from build123d import *

# Parameters (mm, degrees)
SKETCH2_R           = 1.725
SKETCH2_W           = 10
SKETCH2_H           = 20
BOSS_EXTRUDE1_DEPTH = 1.55
FILLET1_R           = 1


with BuildPart() as part:
    # Sketch2 → Boss-Extrude1 (new body)
    # profile 1 of 4: a face of its own
    with BuildSketch(Plane(origin=(0, 0, 0), x_dir=(1, 0, 0), z_dir=(0, 1, 0))):
        Polygon((17.906706977, 15.176380902), (-1.411809549, 10), (-4, 19.659258263), (15.318516526, 24.835639165), align=None)
        with Locations(Location((11.78298262, 18.711914808, 0), (0, 0, 90))):
            Circle(SKETCH2_R, mode=Mode.SUBTRACT)
        with Locations(Location((2.123724357, 16.123724357, 0), (0, 0, 90))):
            Circle(SKETCH2_R, mode=Mode.SUBTRACT)
    # profile 2 of 4: a face of its own
    with BuildSketch(Plane(origin=(0, 0, 0), x_dir=(1, 0, 0), z_dir=(0, 1, 0))):
        Polygon((-1.411809549, 10), (-4, 19.659258263), (-5, 19.39130907), (-5, 10), align=None)
    # profile 3 of 4: a face of its own
    with BuildSketch(Plane(origin=(0, 0, 0), x_dir=(1, 0, 0), z_dir=(0, 1, 0))):
        Rectangle(SKETCH2_W, SKETCH2_H)
        with Locations(Location((0, 5, 0), (0, 0, 90))):
            Circle(SKETCH2_R, mode=Mode.SUBTRACT)
        with Locations(Location((0, -5, 0), (0, 0, 90))):
            Circle(SKETCH2_R, mode=Mode.SUBTRACT)
    # profile 4 of 4: a face of its own
    with BuildSketch(Plane(origin=(0, 0, 0), x_dir=(1, 0, 0), z_dir=(0, 1, 0))):
        Polygon((5, 11.718039191), (-1.411809549, 10), (5, 10), align=None)
    extrude(amount=BOSS_EXTRUDE1_DEPTH)

    # Fillet1
    fillet1_edges = [part.edges().sort_by_distance(p)[0] for p in [
        (-5, 0.775, 10),
        (-5, 0.775, -19.39130907),
        (15.318516526, 0.775, -24.835639165),
        (17.906706977, 0.775, -15.176380902),
        (5, 0.775, -11.718039191),
        (5, 0.775, 10),
    ]]
    fillet(fillet1_edges, radius=FILLET1_R)


solid = part.part
The listing builds one solid part. Answer for the finished solid, in the listing's coordinates (mm). A direction names the side the tool comes from. Give positions to 0.01 mm unless a question says otherwise; leave off trailing zeros. Loops run counter-clockwise (first coordinate to the right, second up) from the corner with the lowest first, then second, coordinate; pieces in that order, holes last. Notation, with made-up numbers: (51.25, 67.5) - (89.25, 67.5) arc R18 ccw to (89.25, 94.5) - close; hole circle Ø9 at (16, 73). An arc over 180 degrees is marked (long way). Use one line per item in the form item = value.
1. Section C-C on x = 2.5 is taken. Give the vertices of the cut face in (y, z).
Calculated:
outline = (0, -21.4) - (1.55, -21.4) - (1.55, -17.81) - (0, -17.81) - close; (0, -14.44) - (1.55, -14.44) - (1.55, 10) - (0, 10) - close
2. Section B-B on x = 0 is taken. Give the vertices of the cut face in (y, z) (3 decimals).
Calculated:
outline = (0, -20.731) - (1.55, -20.731) - (1.55, -6.725) - (0, -6.725) - close; (0, -3.275) - (1.55, -3.275) - (1.55, 3.275) - (0, 3.275) - close; (0, 6.725) - (1.55, 6.725) - (1.55, 10) - (0, 10) - close
3. Find the intervals of material crossed by line 1 along X through (y, z) = (1.2, 5) (3 decimals); line 2 along X through (y, z) = (1.1, -1.5); line 3 along Z through (x, y) = (13.25, 1.3), in increasing order. Write a range as [from, to].
Calculated:
line_1 = [-5, -1.725], [1.725, 5]
line_2 = [-5, 5]
line_3 = [-24.28, -19.62], [-17.8, -13.93]
4. Section A-A on z = -5 is taken. Give the vertices of the cut face in (x, y) (3 decimals).
Calculated:
outline = (-5, 0) - (-1.725, 0) - (-1.725, 1.55) - (-5, 1.55) - close; (1.725, 0) - (5, 0) - (5, 1.55) - (1.725, 1.55) - close
5. Which of the six approach directions +Z, -Z, +X, -X, +Y, -Y give full straight-line access (tool end or side, diameter ignored) to faces 1 (the face through (4, 0, -11)), 2 (the face through (5, 1, -1))?
Calculated:
face_1 = +Z, -Z, +X, -X, -Y
face_2 = +Z, +X, +Y, -Y
6. The mould has two halves that part along X. Classify faces 3 (the face through (0.661, 0.764, -6.593)), 4 (the face through (-5, 1, -5)), 5 (the face through (0, 1, 10)): pulls with the +X half, pulls with the -X half, needs draft (parallel to the pull), parting line crosses it, or undercut.
Calculated:
face_3 = undercut
face_4 = pulls with the -X half
face_5 = needs draft
7. Section D-D on y = 0.9 is taken. Give the vertices of the cut face in (x, z) (3 decimals).
Calculated:
outline = (-5, -18.624) arc R1 ccw to (-4.259, -19.59) - (14.353, -24.577) arc R1 ccw to (15.577, -23.87) - (17.648, -16.142) arc R1 ccw to (16.941, -14.918) - (5.741, -11.917) arc R1 cw to (5, -10.951) - (5, 9) arc R1 ccw to (4, 10) - (-4, 10) arc R1 ccw to (-5, 9) - close; hole circle Ø3.45 at (0, -5); hole circle Ø3.45 at (0, 5); hole circle Ø3.45 at (2.124, -16.124); hole circle Ø3.45 at (11.783, -18.712)
8. Given pin 1 Ø1.5 at (x, z) = (5, -1) entering from -Y; pin 2 Ø3 at (x, z) = (11.78, -18.71) entering from +Y; pin 3 Ø0.8 at (y, z) = (0.5, -4) entering from +X, each flat-ended and moving along its own axis, determine where each tip first touches the part or whether it passes through.
Calculated:
pin_1 = 0
pin_2 = through
pin_3 = 5
